```python
from build123d import *

# Parameters (mm, degrees)
FACE001_W        = 12.25
FACE001_H        = 15.85
FACE001_W_2      = 8
FACE001_H_2      = 8
EXTRUDE001_DEPTH = 4
SKETCH_W         = 15.85
SKETCH_H         = 12.25
EXTRUDE_DEPTH    = 1
FACE002_W        = 12.25
FACE002_H        = 15.85
FACE002_R        = 2.5
EXTRUDE002_DEPTH = 1
FILLET_R         = 0.4


with BuildPart() as extrude001:
    # Face001 → Extrude001 (new body)
    with BuildSketch(Plane(origin=(7.925, 6.125, 1), x_dir=(0, 1, 0), z_dir=(0, 0, 1))):
        Rectangle(FACE001_W, FACE001_H)
        Rectangle(FACE001_W_2, FACE001_H_2, mode=Mode.SUBTRACT)
    extrude(amount=EXTRUDE001_DEPTH)


with BuildPart() as fusion:
    # Sketch → Extrude (new body)
    with BuildSketch(Plane.XY):
        with Locations((7.925, 6.125)):
            Rectangle(SKETCH_W, SKETCH_H)
    extrude(amount=EXTRUDE_DEPTH)

    # Fusion: union Extrude001
    add(extrude001.part)


with BuildPart() as fillet_body:
    # Face002 → Extrude002 (new body)
    with BuildSketch(Plane(origin=(7.925, 6.125, 5), x_dir=(0, 1, 0), z_dir=(0, 0, 1))):
        Rectangle(FACE002_W, FACE002_H)
        Circle(FACE002_R, mode=Mode.SUBTRACT)
    extrude(amount=EXTRUDE002_DEPTH)

    # Fusion001: union Fusion
    add(fusion.part)

    # Fillet
    fillet_edges = [fillet_body.edges().sort_by_distance(p)[0] for p in [
        (15.85, 12.25, 5.5),
        (0, 12.25, 5.5),
        (15.85, 0, 5.5),
        (0, 0, 5.5),
        (15.85, 12.25, 3),
        (0, 12.25, 3),
        (15.85, 0, 3),
        (0, 0, 3),
        (15.85, 12.25, 0.5),
        (0, 12.25, 0.5),
        (15.85, 0, 0.5),
        (0, 0, 0.5),
    ]]
    fillet(fillet_edges, radius=FILLET_R)


solid = fillet_body.part
```
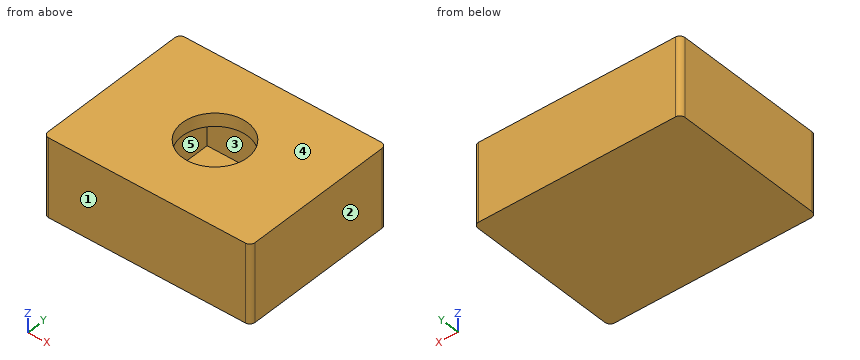
Verification items for the finished model (mm, model axes). Face numbers are marked on the shaded views. A direction names the side the tool comes from. Give positions to 0.01 mm unless a question says otherwise; leave off trailing zeros. Write each loop counter-clockwise with the first axis right and the second up, starting at its lowest first coordinate (ties: lowest second). Pieces come first, ordered by that corner, then holes. Notation, with made-up numbers: (32.25, 56.5) - (62.25, 56.5) arc R24 ccw to (62.25, 79.5) - close; hole circle Ø3 at (88.5, 2.5). An arc over 180 degrees is marked (long way). Put each result on its own line as item: value.
Q1. Set-up check for the marked faces 4 and 5: record each of +Z, -Z, +X, -X, +Y, -Y from which the full face is reachable in a straight line by a thin tool's end or side.
Result:
face 4: +Z, +X, -X, +Y, -Y
face 5: none
Q2. Scan lines: probe 1 along X at (y, z) = (6.5, 2.3) (3 decimals); probe 2 along Y at (x, z) = (7.5, 2.9) (3 decimals); probe 3 along Z at (x, y) = (9, 8.25). Record each from-to range of solid material in increasing order. Write a range as from..to.
Result:
probe 1: 0..3.925, 11.925..15.85
probe 2: 0..2.125, 10.125..12.25
probe 3: 0..1
Q3. Section check B-B on y = 2.5. Record the cut outline in (x, z) (3 decimals), and give its area (3 significant figures).
Result:
outline: (0, 0) - (15.85, 0) - (15.85, 6) - (0, 6) - close; hole (3.925, 1) - (11.925, 1) - (11.925, 5) - (3.925, 5) - close
area: 63.1 mm2
Q4. Mould release check, pull along Y, two halves, no side actions. Record for the marked faces 1, 2 and 3: released by +Y, released by -Y, zero draft, split by the parting line, or undercut.
Result:
face 1: released by -Y
face 2: zero draft
face 3: undercut
Q5. Section check A-A on z = 3.6. Record the cut outline in (x, y) (3 decimals), and give its area (3 significant figures).
Result:
outline: (0, 0.4) arc R0.4 ccw to (0.4, 0) - (15.45, 0) arc R0.4 ccw to (15.85, 0.4) - (15.85, 11.85) arc R0.4 ccw to (15.45, 12.25) - (0.4, 12.25) arc R0.4 ccw to (0, 11.85) - close; hole (3.925, 2.125) - (11.925, 2.125) - (11.925, 10.125) - (3.925, 10.125) - close
area: 130 mm2
Q6. Section check D-D on y = 7. Record the cut outline in (x, z) (3 decimals), and give its area (3 significant figures).
Result:
outline: (0, 0) - (15.85, 0) - (15.85, 6) - (10.267, 6) - (10.267, 5) - (11.925, 5) - (11.925, 1) - (3.925, 1) - (3.925, 5) - (5.583, 5) - (5.583, 6) - (0, 6) - close
area: 58.4 mm2
Q7. Section check C-C on x = 6.25. Record the cut outline in (y, z) (3 decimals), and give its area (3 significant figures).
Result:
outline: (0, 0) - (12.25, 0) - (12.25, 6) - (7.981, 6) - (7.981, 5) - (10.125, 5) - (10.125, 1) - (2.125, 1) - (2.125, 5) - (4.269, 5) - (4.269, 6) - (0, 6) - close
area: 37.8 mm2
